Part model, mm, in its own coordinate system. A direction names the side the tool comes from. Give positions to 0.01 mm unless a question says otherwise; leave off trailing zeros. Order: outer loops, then holes, each group sorted by start corner. A loop starts at its lowest first (then second) coordinate and runs counter-clockwise, first axis right, second up. Notation, with made-up numbers: (88, -36) - (104, -36) arc R26 cw to (104, 2) - close; hole circle Ø3 at (51.25, 83.25). An arc over 180 degrees is marked (long way). Use a Markdown table: item, result. Add a question column.
from build123d import *

# Parameters (mm, degrees)
EXTRUDE_1_DEPTH              = 8
HOLE_WIZARD_M3_1_D           = 3.4
HOLE_WIZARD_M3_1_DEPTH       = 18
HOLE_WIZARD_M3_1_CSINK_D     = 6.3
HOLE_WIZARD_M3_1_CSINK_ANGLE = 90
HOLE_WIZARD_M3_1_2_D         = 2.5
HOLE_WIZARD_M3_1_2_DEPTH     = 18


with BuildPart() as part:
    # 스케치1 → 보스-돌출1 (new body)
    with BuildSketch(Plane.XY):
        with BuildLine():
            Line((1, -13.964240044), (1, -64))
            Line((1, -64), (5, -64))
            Line((5, -64), (19, -25))
            Line((19, -25), (19, 0))
            ThreePointArc((19, 0), (0, 19), (-19, 0))
            Line((-19, 0), (-19, -25))
            Line((-19, -25), (-5, -64))
            Line((-5, -64), (-1, -64))
            Line((-1, -64), (-1, -13.964240044))
            ThreePointArc((-1, -13.964240044), (0, 14), (1, -13.964240044))
        make_face()
    extrude(amount=EXTRUDE_1_DEPTH)

    # Hole Wizard M3 _ _ _ _1
    with Locations(Plane(origin=(19, 0, 0), x_dir=(0, 0, -1), z_dir=(1, 0, 0))):
        with Locations((-4, -18)):
            CounterSinkHole(HOLE_WIZARD_M3_1_D / 2, HOLE_WIZARD_M3_1_CSINK_D / 2, depth=HOLE_WIZARD_M3_1_DEPTH, counter_sink_angle=HOLE_WIZARD_M3_1_CSINK_ANGLE)

    # Hole Wizard M3 _ _1 2
    with Locations(Plane.ZY.offset(19)):
        with Locations((4, -18)):
            Hole(HOLE_WIZARD_M3_1_2_D / 2, depth=HOLE_WIZARD_M3_1_2_DEPTH)


solid = part.part
1. Mould opens along X. For faces 1 (the face through (4, -22, 8)), 2 (the face through (-0.602, 13.987, 3.944)), 3 (the face through (11.902, -44.773, 3.944)) say: released by +X, released by -X, zero draft, split by the parting line, or undercut.
2. Cut at A-A (z = 4). Write the cut outline in (x, y), plus the area to 3 significant figures.
3. Drill centre lines: probe 1 along Z at (x, y) = (11.5, -18); probe 2 along Y at (x, z) = (0, 2.75); probe 3 along X at (y, z) = (-51.5, 6.5). Where is each one in solid material? Low to high. Write a range as [from, to].
4. Cut at D-D (y = -56). Write the cut outline in (x, z), plus the area to 3 significant figures.
5. Cut at C-C (y = -18). Write the cut outline in (x, z).
6. Tool access for faces 4 (the face through (19, -13, 4)), 5 (the face through (1, -39, 4)), 6 (the face through (9.16, -17.49, 5.62)): list every direction of +Z, -Z, +X, -X, +Y, -Y with a clear straight run to the whole face (end or side of a thin tool).
7. Cut at B-B (x = 2). Write the cut outline in (y, z), plus the area to 3 significant figures.
8. Pin check, flat tips, straight feed: P1, Ø3, axis at x = 13, z = 4.5, coming from the +Y side; P2, Ø12, axis at x = -13, y = -34, coming from the -Z side; P3, Ø4, axis at y = -33, z = 4, coming from the +X side; P4, Ø2, axis at y = -18, z = 4, coming from the -X side. Stop position of each tip, or through.
Responses:
| question | item | result |
|---|---|---|
| 1 | face 1 | zero draft |
| 1 | face 2 | undercut |
| 1 | face 3 | released by +X |
| 2 | outline | (-19, -25) - (-5, -64) - (-1, -64) - (-1, -19.25) - (-19, -19.25) - close; (-19, -16.75) - (-1, -16.75) - (-1, -13.96) arc R14 cw (long way) to (1, -13.96) - (1, -16.3) - (17.55, -16.3) - (19, -14.85) - (19, 0) arc R19 ccw to (-19, 0) - close; (1, -64) - (5, -64) - (19, -25) - (19, -21.15) - (17.55, -19.7) - (1, -19.7) - close |
| 2 | area | 1,630 mm² |
| 3 | probe 1 | z = [0, 2.3], [5.7, 8] |
| 3 | probe 2 | y = [14, 19] |
| 3 | probe 3 | x = [-9.49, -1], [1, 9.49] |
| 4 | outline | (-7.87, 0) - (-1, 0) - (-1, 8) - (-7.87, 8) - close; (1, 0) - (7.87, 0) - (7.87, 8) - (1, 8) - close |
| 4 | area | 110 mm² |
| 5 | outline | (-19, 0) - (-1, 0) - (-1, 2.75) - (-19, 2.75) - close; (-19, 5.25) - (-1, 5.25) - (-1, 8) - (-19, 8) - close; (1, 0) - (19, 0) - (19, 0.85) - (17.55, 2.3) - (1, 2.3) - close; (1, 5.7) - (17.55, 5.7) - (19, 7.15) - (19, 8) - (1, 8) - close |
| 6 | face 4 | +Z, -Z, +X, +Y, -Y |
| 6 | face 5 | +Z, -Z, -Y |
| 6 | face 6 | +X |
| 7 | outline | (-64, 0) - (-13.86, 0) - (-13.86, 8) - (-64, 8) - close; (13.86, 0) - (18.89, 0) - (18.89, 8) - (13.86, 8) - close; hole circle Ø3.4 at (-18, 4) |
| 7 | area | 432 mm² |
| 8 | P1 | stops at y = 15.12 |
| 8 | P2 | stops at z = 0 |
| 8 | P3 | stops at x = 16.85 |
| 8 | P4 | passes through |
